from build123d import *

# Parameters (mm, degrees)
ESQUISSE1_W                                = 65
ESQUISSE1_H                                = 56
BOSS_EXTRU_1_DEPTH                         = 6
ESQUISSE4_W                                = 65
ESQUISSE4_H                                = 38
ENL_V_MAT_EXTRU_1_DEPTH                    = 3
ESQUISSE5_W                                = 5
ESQUISSE5_H                                = 5
BOSS_EXTRU_2_DEPTH                         = 25
ESQUISSE6_R                                = 1.1
ENL_V_MAT_EXTRU_2_DEPTH                    = 3
ESQUISSE7_W                                = 4
ESQUISSE7_H                                = 22
ENL_V_MAT_EXTRU_3_DEPTH                    = 50.651283971
SYM_TRIE1_AT_THE_SECOND_PLANE_COPY_1_SKE_W = 5
SYM_TRIE1_AT_THE_SECOND_PLANE_COPY_1_SKE_H = 5
SYM_TRIE1_AT_THE_SECOND_PLANE_COPY_1_DEPTH = 25
SYM_TRIE1_AT_THE_SECOND_PLANE_COPY_2_SKE_R = 1.1
SYM_TRIE1_AT_THE_SECOND_PLANE_COPY_2_DEPTH = 3


with BuildPart() as part:
    # Esquisse1 → Boss.-Extru.1 (new body)
    with BuildSketch(Plane.XY):
        Rectangle(ESQUISSE1_W, ESQUISSE1_H)
    extrude(amount=BOSS_EXTRU_1_DEPTH)

    # Esquisse4 → Enlèv. mat.-Extru.1 (cut)
    with BuildSketch(Plane.XY.offset(6)):
        Rectangle(ESQUISSE4_W, ESQUISSE4_H)
    extrude(amount=-ENL_V_MAT_EXTRU_1_DEPTH, mode=Mode.SUBTRACT)

    # Esquisse5 → Boss.-Extru.2 (add)
    with BuildSketch(Plane(origin=(0, 0, 0), x_dir=(-1, 0, 0), z_dir=(0, 0, -1))):
        with Locations((-30, 25.5)):
            Rectangle(ESQUISSE5_W, ESQUISSE5_H)
    boss_extru_2 = extrude(amount=BOSS_EXTRU_2_DEPTH)

    # Esquisse6 → Enlèv. mat.-Extru.2 (cut)
    with BuildSketch(Plane(origin=(0, 0, -25), x_dir=(-1, 0, 0), z_dir=(0, 0, -1))):
        with Locations((-29, 24.5)):
            Circle(ESQUISSE6_R)
    enl_v_mat_extru_2 = extrude(amount=-ENL_V_MAT_EXTRU_2_DEPTH, mode=Mode.SUBTRACT)

    # Esquisse7 → Enlèv. mat.-Extru.3 (cut, through all)
    with BuildSketch(Plane(origin=(0, 0, 0), x_dir=(-1, 0, 0), z_dir=(0, 0, -1))):
        with Locations((-27.5, 0)):
            Rectangle(ESQUISSE7_W, ESQUISSE7_H)
        with Locations((27.5, 0)):
            Rectangle(ESQUISSE7_W, ESQUISSE7_H)
    extrude(amount=-ENL_V_MAT_EXTRU_3_DEPTH, mode=Mode.SUBTRACT)

    # Symétrie1: Boss.-Extru.2, Enlèv. mat.-Extru.2 across plane
    add(boss_extru_2.mirror(Plane.ZX))
    add(enl_v_mat_extru_2.mirror(Plane.ZX), mode=Mode.SUBTRACT)

    # Symétrie1 at the second plane: Boss.-Extru.2, Enlèv. mat.-Extru.2 across plane
    add(boss_extru_2.mirror(Plane(origin=(0, 0, 0), x_dir=(0, 0, 1), z_dir=(1, 0, 0))))
    add(enl_v_mat_extru_2.mirror(Plane(origin=(0, 0, 0), x_dir=(0, 0, 1), z_dir=(1, 0, 0))), mode=Mode.SUBTRACT)

    # Symétrie1 at the second plane copy 1 ske → Symétrie1 at the second plane copy 1 (add)
    with BuildSketch(Plane(origin=(0, 0, 0), x_dir=(1, 0, 0), z_dir=(0, 0, -1))):
        with Locations((-30, 25.5)):
            Rectangle(SYM_TRIE1_AT_THE_SECOND_PLANE_COPY_1_SKE_W, SYM_TRIE1_AT_THE_SECOND_PLANE_COPY_1_SKE_H)
    extrude(amount=SYM_TRIE1_AT_THE_SECOND_PLANE_COPY_1_DEPTH)

    # Symétrie1 at the second plane copy 2 ske → Symétrie1 at the second plane copy 2 (cut)
    with BuildSketch(Plane(origin=(0, 0, -25), x_dir=(1, 0, 0), z_dir=(0, 0, -1))):
        with Locations((-29, 24.5)):
            Circle(SYM_TRIE1_AT_THE_SECOND_PLANE_COPY_2_SKE_R)
    extrude(amount=-SYM_TRIE1_AT_THE_SECOND_PLANE_COPY_2_DEPTH, mode=Mode.SUBTRACT)


solid = part.part
Work out the finished part from the listing and answer in its coordinate system (mm). A direction names the side the tool comes from. Coordinates: 2 decimals unless noted, no trailing zeros. Write each loop counter-clockwise with the first axis right and the second up, starting at its lowest first coordinate (ties: lowest second). Pieces come first, ordered by that corner, then holes. Notation, with made-up numbers: M 69.5,3 L 77.5,3 A33 ccw 77.5,34 Z; hole C 9,31.25 d11. An arc over 180 degrees is marked long. Write item = value, one per line.
1. The part is cut by section D-D (z = 4). Determine the outline of the cut face in (x, y), then the cut area to 3 significant figures.
Solution:
outline = M -32.5,-28 L 32.5,-28 L 32.5,-19 L -32.5,-19 Z; M -32.5,19 L 32.5,19 L 32.5,28 L -32.5,28 Z
area = 1,170 mm2
2. The part is cut by section B-B (y = 6.5). Determine the outline of the cut face in (x, z), then the cut area to 3 significant figures.
Solution:
outline = M -32.5,0 L -29.5,0 L -29.5,3 L -32.5,3 Z; M -25.5,0 L 25.5,0 L 25.5,3 L -25.5,3 Z; M 29.5,0 L 32.5,0 L 32.5,3 L 29.5,3 Z
area = 171 mm2
3. Determine the mould class of faces 6 (the face through (-29, 25, -22)), 7 (the face through (-32.5, 0, 2)), 8 (the face through (0, -23, 6)) for opening direction X: released by +X, released by -X, zero draft, split by the parting line, or undercut.
Solution:
face_6 = undercut
face_7 = released by -X
face_8 = zero draft
4. The part is cut by section A-A (z = -1). Determine the outline of the cut face in (x, y).
Solution:
outline = M -32.5,-28 L -27.5,-28 L -27.5,-23 L -32.5,-23 Z; M -32.5,23 L -27.5,23 L -27.5,28 L -32.5,28 Z; M 27.5,-28 L 32.5,-28 L 32.5,-23 L 27.5,-23 Z; M 27.5,23 L 32.5,23 L 32.5,28 L 27.5,28 Z
5. Straight lines are drawn through the part: line 1 (Y direction, x = -29, z = -23.1); line 2 (X direction, y = -24.5, z = -23.4); line 3 (X direction, y = 24, z = -23). For each, find the intervals that lie inside material, in ascending order. Write a range as from..to.
Solution:
line_1 = -28..-25.6, -23.4..-23, 23..23.4, 25.6..28
line_2 = -32.5..-30.1, -27.9..-27.5, 27.5..27.9, 30.1..32.5
line_3 = -32.5..-29.98, -28.02..-27.5, 27.5..28.02, 29.98..32.5
6. The part is cut by section C-C (x = 1.5). Determine the outline of the cut face in (y, z), then the cut area to 3 significant figures.
Solution:
outline = M -28,0 L 28,0 L 28,6 L 19,6 L 19,3 L -19,3 L -19,6 L -28,6 Z
area = 222 mm2
7. For faces 1 (the face through (-27, 11, 1)), 2 (the face through (27.5, -25, -12)), 3 (the face through (-30, 23, -12)), 4 (the face through (0, -19, 5)), 5 (the face through (-29, -25, -22)), determine the directions among +Z, -Z, +X, -X, +Y, -Y from which every point of the face is accessible in a straight line to the end or side of a thin tool.
Solution:
face_1 = +Z, -Z
face_2 = -Z, +Y, -Y
face_3 = -Z, +X, -X
face_4 = +Z, +X, -X
face_5 = -Z
8. Flat-ended cylindrical pins translate along their axes: pin 1 (2 mm diameter, centred on x = 20, y = -7, fed in from +Z); pin 2 (2 mm diameter, centred on x = 17, y = 4.5, fed in from -Z); pin 3 (0.7 mm diameter, centred on x = 29, y = -25, fed in from -Z); pin 4 (10 mm diameter, centred on y = 21, z = -18, fed in from +X). Find the tip coordinate at first contact, or state that the pin passes through.
Solution:
pin_1 = 3
pin_2 = 0
pin_3 = -22
pin_4 = 32.5
